Check sheet for the modelled part. Datum: model origin and axes. Units: mm. A direction names the side the tool comes from. Round coordinates to 2 decimals unless told otherwise and drop trailing zeros. Loops run counter-clockwise (first coordinate to the right, second up) from the corner with the lowest first, then second, coordinate; pieces in that order, holes last. Notation, with made-up numbers: (-29, -31) - (22, -31) arc R20 cw to (22, -13) - close; hole circle Ø2 at (19.25, -27). An arc over 180 degrees is marked (long way). Put each result on its own line as item: value. Start each with the question number.
Item 1: Section check C-C, the plane y = 2.5. Record the cut outline in (x, z) (3 decimals).
Item 2: Section check A-A, the plane x = 0. Give the number of separate pieces and of enclosed holes in the cut face, and give its area (3 significant figures).
Item 3: Material ranges on line 1 along X through (y, z) = (-4.45, -32.65); line 2 along Z through (x, y) = (-26, -12); line 3 along Y through (x, z) = (14.5, -24.5), recorded low to high.
Item 4: Section check B-B, the plane z = -4.5. Record the cut outline in (x, y) (1 decimal), and give its area (3 significant figures).
Item 5: Gauge pin test, flat ends, axial feed: pin 1 Ø10.5 at (x, y) = (3, -1.5) entering from +Z; pin 2 Ø3 at (x, y) = (-12, -13.26) entering from +Z; pin 3 Ø3 at (y, z) = (-5.5, -3.5) entering from +X; pin 4 Ø9 at (x, z) = (4, -36) entering from -Y. Record the tip position at first contact, or that the pin passes through.
Item 6: Tool access check on faces 1 (the flat face through (-13.263, 0.067, -13.36)), 2 (the cylindrical face through (0.4, 4.27, -41.64)), 3 (the cylindrical face through (-0.264, -1.228, -38.644)). Record the directions out of +Z, -Z, +X, -X, +Y, -Y that give a thin tool (end or side, any length) a straight path to the whole face; none if there is none.
Item 7: Draft check along X on faces 4 (the flat face through (-1.9, -3.762, -26.8)), 5 (the flat face through (20.67, -4.26, -27.64)), 6 (the flat face through (-20.795, 0.053, -28.299)). Enter one of: pulls with the +X half, pulls with the -X half, needs draft (parallel to the pull), parting line crosses it, or undercut.
Item 8: Section check D-D, the plane y = -8.25. Record the cut outline in (x, z) (3 decimals).
from build123d import *

# Parameters (mm, degrees)
SKETCH1_R           = 5
BOSS_EXTRUDE1_DEPTH = 4.7625
SKETCH2_R           = 9
SKETCH2_R_2         = 6
CUT_EXTRUDE1_DEPTH  = 1
FILLET1_R           = 5
CUT_EXTRUDE2_START  = -6
SKETCH3_R           = 6
CUT_EXTRUDE2_DEPTH  = 6
SKETCH4_R           = 2.5
BOSS_EXTRUDE2_DEPTH = 6.35
CHAMFER3_SIZE       = 1


with BuildPart() as part:
    # Sketch1 → Boss-Extrude1 (new, symmetric)
    with BuildSketch(Plane(origin=(0, 0, 0), x_dir=(1, 0, 0), z_dir=(0, 1, 0))):
        with BuildLine():
            Line((-30.675, 0), (-15.675, 0))
            Line((-15.675, 0), (-15.675, 10.154547549))
            Line((-15.675, 10.154547549), (-9.282686693, 18.65))
            Line((-9.282686693, 18.65), (9.282686693, 18.65))
            Line((9.282686693, 18.65), (15.675, 10.154547549))
            Line((15.675, 10.154547549), (15.675, 0))
            Line((15.675, 0), (30.675, 0))
            Line((30.675, 0), (30.675, 15.167545938))
            Line((30.675, 15.167545938), (11.186887419, 41.067455071))
            ThreePointArc((11.186887419, 41.067455071), (0, 46.65), (-11.186887419, 41.067455071))
            Line((-11.186887419, 41.067455071), (-30.675, 15.167545938))
            Line((-30.675, 15.167545938), (-30.675, 0))
        make_face()
        with Locations(Location((0, 32.65, 0), (0, 0, 90))):
            Circle(SKETCH1_R, mode=Mode.SUBTRACT)
    extrude(amount=BOSS_EXTRUDE1_DEPTH, both=True)

    # Sketch2 → Cut-Extrude1 (cut)
    with BuildSketch(Plane(origin=(0, 4.7625, 0), x_dir=(1, 0, 0), z_dir=(0, 1, 0))):
        with Locations(Location((0, 32.65, 0), (0, 0, 270))):
            Circle(SKETCH2_R)
        with Locations(Location((0, 32.65, 0), (0, 0, 270))):
            Circle(SKETCH2_R_2, mode=Mode.SUBTRACT)
    cut_extrude1 = extrude(amount=-CUT_EXTRUDE1_DEPTH, mode=Mode.SUBTRACT)

    # Fillet1
    fillet1_edges = [part.edges().sort_by_distance(p)[0] for p in [
        (9.282686693, 0, -18.65),
        (-9.282686693, 0, -18.65),
    ]]
    fillet(fillet1_edges, radius=FILLET1_R)

    # Sketch3 → Cut-Extrude2 (cut)
    with BuildSketch(Plane.XZ.offset(4.7625).offset(CUT_EXTRUDE2_START)):
        with Locations(Location((0, -32.65, 0), (0, 0, 90))):
            Circle(SKETCH3_R)
    extrude(amount=CUT_EXTRUDE2_DEPTH, mode=Mode.SUBTRACT)

    # Mirror2: Cut-Extrude1 across plane
    add(cut_extrude1.mirror(Plane.ZX), mode=Mode.SUBTRACT)

    # Sketch4 → Boss-Extrude2 (add)
    with BuildSketch(Plane.XY):
        with BuildLine():
            Line((-16.675, -23.7375), (16.675, -23.7375))
            ThreePointArc((16.675, -23.7375), (26.574494937, -19.636994937), (30.675, -9.7375))
            Line((30.675, -9.7375), (30.675, 4.7625))
            Line((30.675, 4.7625), (15.675, 4.7625))
            Line((15.675, 4.7625), (15.675, -4.7625))
            ThreePointArc((15.675, -4.7625), (0, -12.392034951), (-15.675, -4.7625))
            Line((-15.675, -4.7625), (-15.675, 4.7625))
            Line((-15.675, 4.7625), (-30.675, 4.7625))
            Line((-30.675, 4.7625), (-30.675, -9.7375))
            ThreePointArc((-30.675, -9.7375), (-26.574494937, -19.636994937), (-16.675, -23.7375))
        make_face()
        with Locations((-12, -13.259609691)):
            Circle(SKETCH4_R, mode=Mode.SUBTRACT)
        with Locations((12, -13.259609691)):
            Circle(SKETCH4_R, mode=Mode.SUBTRACT)
    extrude(amount=BOSS_EXTRUDE2_DEPTH)

    # Chamfer3
    chamfer3_edges = [part.edges().sort_by_distance(p)[0] for p in [
        (-20.93094371, -4.7625, -28.117500504),
        (0, -4.7625, -46.65),
        (20.93094371, -4.7625, -28.117500504),
        (30.675, -4.7625, -7.583772969),
        (-30.675, -4.7625, -7.583772969),
        (30.675, 4.7625, -4.408772969),
        (20.93094371, 4.7625, -28.117500504),
        (0, 4.7625, -46.65),
        (-20.93094371, 4.7625, -28.117500504),
        (-30.675, 4.7625, -4.408772969),
        (-30.675, -7.25, 0),
        (-26.574494937, -19.636994937, 0),
        (0, -23.7375, 0),
        (26.574494937, -19.636994937, 0),
        (30.675, -7.25, 0),
    ]]
    chamfer(chamfer3_edges, length=CHAMFER3_SIZE)


solid = part.part
Check result:
1. outline: (-30.675, -15.168) - (-11.187, -41.067) arc R14 ccw to (11.187, -41.067) - (30.675, -15.168) - (30.675, 6.35) - (15.675, 6.35) - (15.675, -10.155) - (10.783, -16.656) arc R5 cw to (6.788, -18.65) - (-6.788, -18.65) arc R5 cw to (-10.783, -16.656) - (-15.675, -10.155) - (-15.675, 6.35) - (-30.675, 6.35) - close; hole circle Ø10 at (0, -32.65)
2. separate pieces: 3
2. enclosed holes: 0
2. area: 218 mm²
3. line 1: -16.66 to -9, 9 to 16.66
3. line 2: 0 to 6.35
3. line 3: -4.76 to 4.76
4. outline: (-30.7, -3.8) - (-29.7, -4.8) - (-15.7, -4.8) - (-15.7, 4.8) - (-29.7, 4.8) - (-30.7, 3.8) - close; (15.7, -4.8) - (29.7, -4.8) - (30.7, -3.8) - (30.7, 3.8) - (29.7, 4.8) - (15.7, 4.8) - close
4. area: 284 mm²
5. pin 1: z = -18.43
5. pin 2: through
5. pin 3: x = 30.44
5. pin 4: y = -4.76
6. face 1: +Z, +Y, -Y
6. face 2: +Y
6. face 3: -Y
7. face 4: undercut
7. face 5: pulls with the +X half
7. face 6: pulls with the -X half
8. outline: (-30.675, 1) - (-29.675, 0) - (-12.159, 0) - (-12.159, 6.35) - (-30.675, 6.35) - close; (12.159, 0) - (29.675, 0) - (30.675, 1) - (30.675, 6.35) - (12.159, 6.35) - close
